Geometry: see drawing. Coordinates: mm, zero at the bounding-box minimum. A direction names the side the tool comes from. Round coordinates to 2 decimals unless told otherwise and drop trailing zeros. Order: outer loops, then holes, each group sorted by start corner. A loop starts at its lowest first (then second) coordinate and runs counter-clockwise, first axis right, second up. Notation, with made-up numbers: (34.25, -36) -> (54.25, -36) arc R23 cw to (54.25, -18) -> close; hole circle Ø3 at (24.25, 47). An arc over 180 degrees is marked (long way). Use a Markdown table: item, result.
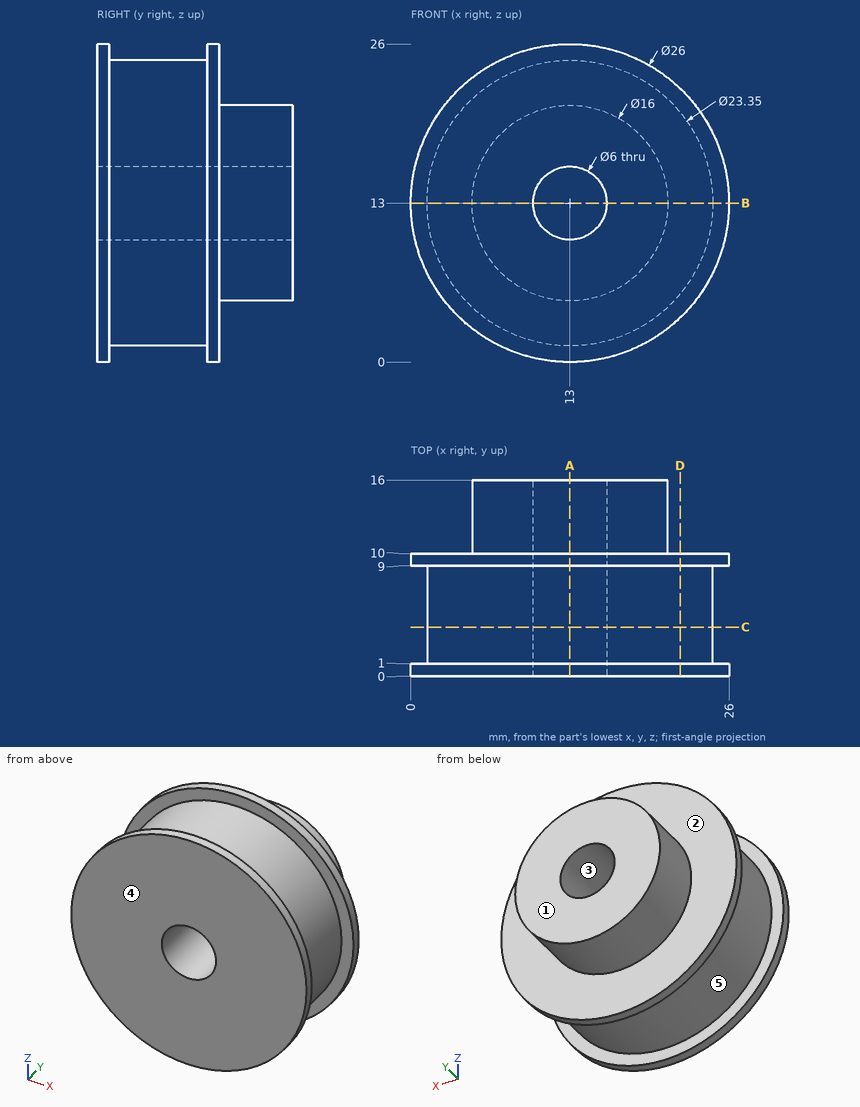
1) Cut plane B-B on z = 13. Return loops of the section in (x, y) (3 decimals).
Answer key:
| item | result |
|---|---|
| outline | (0, 0) -> (10, 0) -> (10, 16) -> (5, 16) -> (5, 10) -> (0, 10) -> (0, 9) -> (1.325, 9) -> (1.325, 1) -> (0, 1) -> close; (16, 0) -> (26, 0) -> (26, 1) -> (24.675, 1) -> (24.675, 9) -> (26, 9) -> (26, 10) -> (21, 10) -> (21, 16) -> (16, 16) -> close |
2) Cut plane C-C on y = 4. Return loops of the section in (x, z) (3 decimals).
Answer key:
| item | result |
|---|---|
| outline | circle Ø23.35 at (13, 13); hole circle Ø6 at (13, 13) |
3) Cut plane D-D on x = 22. Return loops of the section in (y, z), and give its area (3 significant figures).
Answer key:
| item | result |
|---|---|
| outline | (0, 3.62) -> (1, 3.62) -> (1, 5.56) -> (9, 5.56) -> (9, 3.62) -> (10, 3.62) -> (10, 22.38) -> (9, 22.38) -> (9, 20.44) -> (1, 20.44) -> (1, 22.38) -> (0, 22.38) -> close |
| area | 157 mm^2 |
4) Ray query, probe 1 along X at (y, z) = (7.75, 13) (3 decimals); probe 2 along Z at (x, y) = (13, 11). Return the intervals inside material, ascending.
Answer key:
| item | result |
|---|---|
| probe 1 | x = 1.325 to 10, 16 to 24.675 |
| probe 2 | z = 5 to 10, 16 to 21 |
5) Set-up query: the marked faces 1 and 2. Return all of +Z, -Z, +X, -X, +Y, -Y with unobstructed straight access to the full face (end or side cutting, diameter ignored); none if empty.
Answer key:
| item | result |
|---|---|
| face 1 | +Z, -Z, +X, -X, +Y |
| face 2 | +Y |
6) Contact query for flat-ended pins moving along their axis: P1, Ø1.5, axis at y = 3, z = 11, coming from the -X side; P2, Ø5, axis at y = 9.5, z = 19.5, coming from the -X side; P3, Ø8, axis at x = 3.5, y = 6, coming from the +Z side. Output: stop coordinate, or through.
Answer key:
| item | result |
|---|---|
| P1 | stops at x = 1.39 |
| P2 | stops at x = 0.63 |
| P3 | stops at z = 24.05 |
7) Cut plane A-A on x = 13. Return loops of the section in (y, z) (3 decimals).
Answer key:
| item | result |
|---|---|
| outline | (0, 0) -> (1, 0) -> (1, 1.325) -> (9, 1.325) -> (9, 0) -> (10, 0) -> (10, 5) -> (16, 5) -> (16, 10) -> (0, 10) -> close; (0, 16) -> (16, 16) -> (16, 21) -> (10, 21) -> (10, 26) -> (9, 26) -> (9, 24.675) -> (1, 24.675) -> (1, 26) -> (0, 26) -> close |
8) Draft query along Z for the marked faces 3, 4 and 5. Return one class per face: released by +Z, released by -Z, zero draft, split by the parting line, or undercut.
Answer key:
| item | result |
|---|---|
| face 3 | undercut |
| face 4 | zero draft |
| face 5 | split by the parting line |
